```python
from build123d import *

# Parameters (mm, degrees)
BOSS_EXTRUDE1_DEPTH = 3.175
SKETCH1_8_R         = 3.999992
CUT_EXTRUDE1_DEPTH  = 20.701
SKETCH1_9_R         = 3.999992
CUT_EXTRUDE2_DEPTH  = 19.431
CUT_EXTRUDE8_DEPTH  = 20.193
FILLET1_R           = 12.7
CUT_EXTRUDE9_DEPTH  = 126.238


with BuildPart() as part:
    # Sketch1 → Boss-Extrude1 (new body)
    with BuildSketch(Plane.XY.offset(1577.629912845)):
        with BuildLine():
            Line((50.788624607, 668.00159627), (50.788624607, 617.20159627))
            Line((50.788624607, 617.20159627), (-50.788624607, 617.20159627))
            Line((-50.788624607, 617.20159627), (-50.788624607, 668.00159627))
            ThreePointArc((-50.788624607, 668.00159627), (-47.580641699, 674.404695353), (-40.531332209, 675.668842459))
            Line((-40.531332209, 675.668842459), (0, 663.705728602))
            Line((0, 663.705728602), (40.531332209, 675.668842459))
            ThreePointArc((40.531332209, 675.668842459), (47.580641699, 674.404695353), (50.788624607, 668.00159627))
        make_face()
    extrude(amount=BOSS_EXTRUDE1_DEPTH)

    # Sketch1<8> → Cut-Extrude1 (cut)
    with BuildSketch(Plane.XY.offset(1577.629912845)):
        with Locations((42.794374999, 668.00159627)):
            Circle(SKETCH1_8_R)
    extrude(amount=CUT_EXTRUDE1_DEPTH, mode=Mode.SUBTRACT)

    # Sketch1<9> → Cut-Extrude2 (cut)
    with BuildSketch(Plane.XY.offset(1577.629912845)):
        with Locations((-42.794374999, 668.00159627)):
            Circle(SKETCH1_9_R)
    extrude(amount=CUT_EXTRUDE2_DEPTH, mode=Mode.SUBTRACT)

    # Sketch1<17> → Cut-Extrude8 (cut)
    with BuildSketch(Plane.XY.offset(1577.629912845)):
        with BuildLine():
            Line((13.57510941, 635.333202119), (27.654813941, 657.899286932))
            ThreePointArc((27.654813941, 657.899286932), (27.495220576, 662.168612345), (23.471836113, 663.605618605))
            Line((23.471836113, 663.605618605), (9.392131582, 659.978176021))
            ThreePointArc((9.392131582, 659.978176021), (7.331231426, 658.6225908), (6.532685397, 656.288657429))
            Line((6.532685397, 656.288657429), (6.532685397, 637.350015199))
            ThreePointArc((6.532685397, 637.350015199), (9.293741997, 633.687254253), (13.57510941, 635.333202119))
        make_face()
        with BuildLine():
            Line((38.399954792, 655.927224031), (24.340132355, 638.265442375))
            ThreePointArc((24.340132355, 638.265442375), (23.94914071, 634.774942338), (26.92351994, 632.906913117))
            Line((26.92351994, 632.906913117), (40.983342377, 632.906913117))
            ThreePointArc((40.983342377, 632.906913117), (43.318208968, 633.874046526), (44.285342377, 636.208913117))
            Line((44.285342377, 636.208913117), (44.285342377, 653.870694774))
            ThreePointArc((44.285342377, 653.870694774), (42.072575638, 656.987868959), (38.399954792, 655.927224031))
        make_face()
        with BuildLine():
            Line((-44.285342377, 636.208913117), (-44.285342377, 653.870694774))
            ThreePointArc((-44.285342377, 653.870694774), (-42.072575638, 656.987868959), (-38.399954792, 655.927224031))
            Line((-38.399954792, 655.927224031), (-24.340132355, 638.265442375))
            ThreePointArc((-24.340132355, 638.265442375), (-23.94914071, 634.774942338), (-26.92351994, 632.906913117))
            Line((-26.92351994, 632.906913117), (-40.983342377, 632.906913117))
            ThreePointArc((-40.983342377, 632.906913117), (-43.318208968, 633.874046526), (-44.285342377, 636.208913117))
        make_face()
        with BuildLine():
            Line((-6.532685397, 656.288657429), (-6.532685397, 637.350015199))
            ThreePointArc((-6.532685397, 637.350015199), (-9.293741997, 633.687254253), (-13.57510941, 635.333202119))
            Line((-13.57510941, 635.333202119), (-27.654813941, 657.899286932))
            ThreePointArc((-27.654813941, 657.899286932), (-27.495220576, 662.168612345), (-23.471836113, 663.605618605))
            Line((-23.471836113, 663.605618605), (-9.392131582, 659.978176021))
            ThreePointArc((-9.392131582, 659.978176021), (-7.331231426, 658.6225908), (-6.532685397, 656.288657429))
        make_face()
    extrude(amount=CUT_EXTRUDE8_DEPTH, mode=Mode.SUBTRACT)

    # Fillet1
    fillet1_edges = [part.edges().sort_by_distance(p)[0] for p in [
        (0, 663.705728602, 1579.217412845),
    ]]
    fillet(fillet1_edges, radius=FILLET1_R)

    # Sketch5 → Cut-Extrude9 (cut)
    with BuildSketch(Plane(origin=(50.788624607, 0, 0), x_dir=(0, 0, -1), z_dir=(1, 0, 0))):
        Polygon((-1577.636028368, 625.473682851), (-1580.804912845, 622.730103166), (-1584.510921517, 619.521488216), (-1584.510921517, 612.304065089), (-1576.030251426, 612.304065089), (-1576.030251426, 626.863944008), align=None)
    extrude(amount=-CUT_EXTRUDE9_DEPTH, mode=Mode.SUBTRACT)


solid = part.part
```
Verification items for the finished model (mm, model axes). A direction names the side the tool comes from. Give positions to 0.01 mm unless a question says otherwise; leave off trailing zeros. Order: outer loops, then holes, each group sorted by start corner. A loop starts at its lowest first (then second) coordinate and runs counter-clockwise, first axis right, second up. Notation, with made-up numbers: (-4, -4) -> (41, -4) arc R28 cw to (41, 21) -> close; hole circle Ø11 at (-36.75, 40). An arc over 180 degrees is marked (long way). Use a Markdown table: item, result.
1) Mould release check, pull along Y, two halves, no side actions. Record for faces 4 (the cylindrical face through (43.292, 633.849, 1579.195)), 5 (the cylindrical face through (42.274, 671.968, 1579.195)), 6 (the flat face through (1, 644, 1580.805)), 7 (the flat face through (-22.322, 670.294, 1579.195)): pulls with the +Y half, pulls with the -Y half, needs draft (parallel to the pull), parting line crosses it, or undercut.
Results:
| item | result |
|---|---|
| face 4 | undercut |
| face 5 | undercut |
| face 6 | needs draft |
| face 7 | pulls with the +Y half |
2) Tool access check on faces 1 (the flat face through (1, 651, 1577.63)), 2 (the cylindrical face through (-42.126, 656.969, 1579.195)), 3 (the flat face through (21.8, 670.14, 1579.2)). Record the directions out of +Z, -Z, +X, -X, +Y, -Y that give a thin tool (end or side, any length) a straight path to the whole face; none if there is none.
Results:
| item | result |
|---|---|
| face 1 | -Z, +X, -X, +Y, -Y |
| face 2 | +Z, -Z |
| face 3 | +Z, -Z, +Y |
3) Section check D-D, the plane y = 659. Record the boundary of the cut face in (x, z).
Results:
| item | result |
|---|---|
| outline | (-50.79, 1577.63) -> (-28.12, 1577.63) -> (-28.12, 1580.8) -> (-50.79, 1580.8) -> close; (-7.67, 1577.63) -> (7.67, 1577.63) -> (7.67, 1580.8) -> (-7.67, 1580.8) -> close; (28.12, 1577.63) -> (50.79, 1577.63) -> (50.79, 1580.8) -> (28.12, 1580.8) -> close |
4) Section check A-A, the plane x = 11.5. Record the boundary of the cut face in (y, z), then the cut area to 3 significant figures.
Results:
| item | result |
|---|---|
| outline | (622.73, 1580.8) -> (625.48, 1577.63) -> (633.72, 1577.63) -> (633.72, 1580.8) -> close; (660.52, 1577.63) -> (667.1, 1577.63) -> (667.1, 1580.8) -> (660.52, 1580.8) -> close |
| area | 51.4 mm² |
5) Depth check by flat-ended pin: pin 1 Ø1 at (x, z) = (30.5, 1578.5) entering from -Y; pin 2 Ø1 at (x, z) = (-33, 1579.5) entering from +Y; pin 3 Ø1.5 at (x, z) = (-29, 1579.5) entering from +Y. Enter the tip coordinate at first touch or a pass-through.
Results:
| item | result |
|---|---|
| pin 1 | y = 624.29 |
| pin 2 | y = 673.59 |
| pin 3 | y = 672.49 |
6) Section check B-B, the plane z = 1578.15. Give the number of separate pieces and of enclosed holes in the cut face, then the cut area to 3 significant figures.
Results:
| item | result |
|---|---|
| separate pieces | 1 |
| enclosed holes | 6 |
| area | 3,050 mm² |
7) Section check C-C, the plane y = 649. Record the boundary of the cut face in (x, z).
Results:
| item | result |
|---|---|
| outline | (-50.79, 1577.63) -> (-44.29, 1577.63) -> (-44.29, 1580.8) -> (-50.79, 1580.8) -> close; (-32.89, 1577.63) -> (-22.1, 1577.63) -> (-22.1, 1580.8) -> (-32.89, 1580.8) -> close; (-6.53, 1577.63) -> (6.53, 1577.63) -> (6.53, 1580.8) -> (-6.53, 1580.8) -> close; (22.1, 1577.63) -> (32.89, 1577.63) -> (32.89, 1580.8) -> (22.1, 1580.8) -> close; (44.29, 1577.63) -> (50.79, 1577.63) -> (50.79, 1580.8) -> (44.29, 1580.8) -> close |
8) Material ranges on probe 1 along Y at (x, z) = (25, 1579.45); probe 2 along X at (y, z) = (643.5, 1579.7); probe 3 along X at (y, z) = (639, 1580), recorded low to high.
Results:
| item | result |
|---|---|
| probe 1 | 623.9 to 633.53, 639.09 to 653.64, 663.68 to 671.08 |
| probe 2 | -50.79 to -44.29, -28.51 to -18.67, -6.53 to 6.53, 18.67 to 28.51, 44.29 to 50.79 |
| probe 3 | -50.79 to -44.29, -24.92 to -15.86, -6.53 to 6.53, 15.86 to 24.92, 44.29 to 50.79 |
